Read the model definition and answer for the solid it produces. Units are mm, in the model's axes. Give positions to 0.01 mm unless a question says otherwise; leave off trailing zeros. Write each loop counter-clockwise with the first axis right and the second up, starting at its lowest first coordinate (ties: lowest second). Pieces come first, ordered by that corner, then holes. Notation, with made-up numbers: M 24,80 L 48,80 A18 cw 48,102 Z; hole C 45.5,25 d6. An arc over 180 degrees is marked long. Use a Markdown table: item, result. Add a question column.
Item 1: A cutting plane is placed at B-B on x = 72.5. Determine the outline of the cut face in (y, z).
Item 2: A cutting plane is placed at A-A on y = 6.5. Determine the outline of the cut face in (x, z), then the cut area to 3 significant figures.
Item 3: Given P1, Ø3.5, axis at x = -258, z = 0, coming from the +Y side, flat-ended and moving along its own axis, determine where the tip first touches the part or whether it passes through.
Item 4: Consider probe 1 along Z at (x, y) = (290, 1.1); probe 2 along X at (y, z) = (9.5, -5.5); probe 3 along X at (y, z) = (8.25, 15). Determine where each line is inside the solid, lowest interval first. Write a range as [from, to].
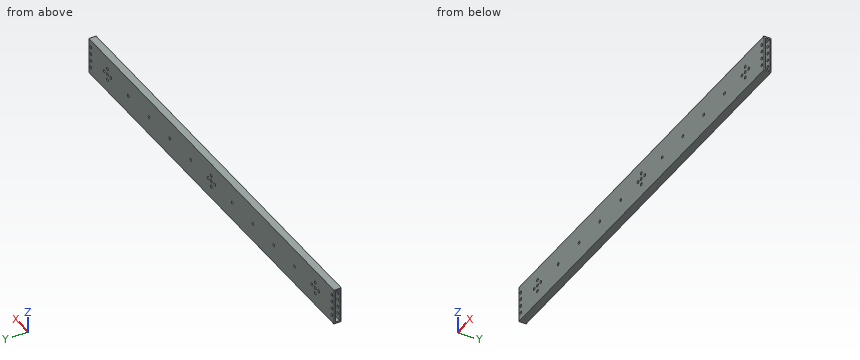
from build123d import *

# Parameters (mm, degrees)
SKETCH_1_W          = 700
SKETCH_1_H          = 50
EXTRUDE_1_DEPTH     = 10
SKETCH_2_R          = 2.05
CUT_EXTRUDE_2_DEPTH = 352.034186369
SKETCH_3_R          = 2.05
CUT_EXTRUDE_3_DEPTH = 352.034186369
SKETCH_4_W          = 46
SKETCH_4_H          = 6
CUT_EXTRUDE_4_DEPTH = 701.51766573
SKETCH_6_W          = 50
SKETCH_6_H          = 10
CUT_EXTRUDE_6_DEPTH = 5
SKETCH_7_R          = 2
CUT_EXTRUDE_7_DEPTH = 347.04912946
SKETCH_8_W          = 50
SKETCH_8_H          = 10
CUT_EXTRUDE_8_DEPTH = 50


with BuildPart() as part:
    # 草图1 → 凸台-拉伸1 (new body)
    with BuildSketch(Plane(origin=(0, 0, 0), x_dir=(1, 0, 0), z_dir=(0, 1, 0))):
        Rectangle(SKETCH_1_W, SKETCH_1_H)
    extrude(amount=EXTRUDE_1_DEPTH)

    # 草图2 → 切除-拉伸2 (cut, through all)
    with BuildSketch(Plane(origin=(0, 10, 0), x_dir=(1, 0, 0), z_dir=(0, 1, 0))):
        with Locations(Location((-300, 0, 0), (0, 0, 270))):
            Circle(SKETCH_2_R)
        with Locations(Location((-250, 0, 0), (0, 0, 270))):
            Circle(SKETCH_2_R)
        with Locations(Location((-200, 0, 0), (0, 0, 270))):
            Circle(SKETCH_2_R)
        with Locations(Location((-150, 0, 0), (0, 0, 270))):
            Circle(SKETCH_2_R)
        with Locations(Location((-100, 0, 0), (0, 0, 270))):
            Circle(SKETCH_2_R)
        with Locations(Location((-50, 0, 0), (0, 0, 270))):
            Circle(SKETCH_2_R)
        with Locations(Location((0, 0, 0), (0, 0, 270))):
            Circle(SKETCH_2_R)
        with Locations(Location((50, 0, 0), (0, 0, 270))):
            Circle(SKETCH_2_R)
        with Locations(Location((100, 0, 0), (0, 0, 270))):
            Circle(SKETCH_2_R)
        with Locations(Location((150, 0, 0), (0, 0, 270))):
            Circle(SKETCH_2_R)
        with Locations(Location((200, 0, 0), (0, 0, 270))):
            Circle(SKETCH_2_R)
        with Locations(Location((250, 0, 0), (0, 0, 270))):
            Circle(SKETCH_2_R)
        with Locations(Location((300, 0, 0), (0, 0, 270))):
            Circle(SKETCH_2_R)
    extrude(amount=-CUT_EXTRUDE_2_DEPTH, mode=Mode.SUBTRACT)

    # 草图3 → 切除-拉伸3 (cut, through all)
    with BuildSketch(Plane(origin=(0, 10, 0), x_dir=(1, 0, 0), z_dir=(0, 1, 0))):
        with Locations(Location((-242, 0, 0), (0, 0, 270))):
            Circle(SKETCH_3_R)
        with Locations(Location((-258, 0, 0), (0, 0, 270))):
            Circle(SKETCH_3_R)
        with Locations(Location((-8, 0, 0), (0, 0, 270))):
            Circle(SKETCH_3_R)
        with Locations(Location((8, 0, 0), (0, 0, 270))):
            Circle(SKETCH_3_R)
        with Locations(Location((242, 0, 0), (0, 0, 270))):
            Circle(SKETCH_3_R)
        with Locations(Location((258, 0, 0), (0, 0, 270))):
            Circle(SKETCH_3_R)
        with Locations(Location((-250, 8, 0), (0, 0, 270))):
            Circle(SKETCH_3_R)
        with Locations(Location((-250, -8, 0), (0, 0, 270))):
            Circle(SKETCH_3_R)
        with Locations(Location((0, 8, 0), (0, 0, 270))):
            Circle(SKETCH_3_R)
        with Locations(Location((0, -8, 0), (0, 0, 270))):
            Circle(SKETCH_3_R)
        with Locations(Location((250, 8, 0), (0, 0, 270))):
            Circle(SKETCH_3_R)
        with Locations(Location((250, -8, 0), (0, 0, 270))):
            Circle(SKETCH_3_R)
    extrude(amount=-CUT_EXTRUDE_3_DEPTH, mode=Mode.SUBTRACT)

    # 草图4 → 切除-拉伸4 (cut, through all)
    with BuildSketch(Plane.ZY.offset(350)):
        with Locations((0, 5)):
            Rectangle(SKETCH_4_W, SKETCH_4_H)
    extrude(amount=-CUT_EXTRUDE_4_DEPTH, mode=Mode.SUBTRACT)

    # 草图6 → 切除-拉伸6 (cut)
    with BuildSketch(Plane(origin=(350, 0, 0), x_dir=(0, 0, -1), z_dir=(1, 0, 0))):
        with Locations((0, 5)):
            Rectangle(SKETCH_6_W, SKETCH_6_H)
    cut_extrude_6 = extrude(amount=-CUT_EXTRUDE_6_DEPTH, mode=Mode.SUBTRACT)

    # 镜向1: 切除-拉伸6 across plane
    add(cut_extrude_6.mirror(Plane(origin=(0, 0, 0), x_dir=(0, 0, 1), z_dir=(1, 0, 0))), mode=Mode.SUBTRACT)

    # 草图7 → 切除-拉伸7 (cut, through all)
    with BuildSketch(Plane(origin=(0, 10, 0), x_dir=(1, 0, 0), z_dir=(0, 1, 0))):
        with Locations(Location((340, 15, 0), (0, 0, 270))):
            Circle(SKETCH_7_R)
        with Locations(Location((340, 5, 0), (0, 0, 270))):
            Circle(SKETCH_7_R)
        with Locations(Location((340, -5, 0), (0, 0, 270))):
            Circle(SKETCH_7_R)
        with Locations(Location((340, -15, 0), (0, 0, 270))):
            Circle(SKETCH_7_R)
        with Locations(Location((290, 5, 0), (0, 0, 270))):
            Circle(SKETCH_7_R)
        with Locations(Location((290, 15, 0), (0, 0, 270))):
            Circle(SKETCH_7_R)
        with Locations(Location((290, -5, 0), (0, 0, 270))):
            Circle(SKETCH_7_R)
        with Locations(Location((290, -15, 0), (0, 0, 270))):
            Circle(SKETCH_7_R)
    cut_extrude_7 = extrude(amount=-CUT_EXTRUDE_7_DEPTH, mode=Mode.SUBTRACT)

    # 镜向2: 切除-拉伸7 across plane
    add(cut_extrude_7.mirror(Plane(origin=(0, 0, 0), x_dir=(0, 0, 1), z_dir=(1, 0, 0))), mode=Mode.SUBTRACT)

    # 草图8 → 切除-拉伸8 (cut)
    with BuildSketch(Plane(origin=(345, 0, 0), x_dir=(0, 0, -1), z_dir=(1, 0, 0))):
        with Locations((0, 5)):
            Rectangle(SKETCH_8_W, SKETCH_8_H)
    cut_extrude_8 = extrude(amount=-CUT_EXTRUDE_8_DEPTH, mode=Mode.SUBTRACT)

    # 镜向3: 切除-拉伸8 across plane
    add(cut_extrude_8.mirror(Plane(origin=(0, 0, 0), x_dir=(0, 0, 1), z_dir=(1, 0, 0))), mode=Mode.SUBTRACT)


solid = part.part
Filled in:
| question | item | result |
|---|---|---|
| 1 | outline | M 0,-25 L 10,-25 L 10,25 L 0,25 Z; hole M 2,-23 L 8,-23 L 8,23 L 2,23 Z |
| 2 | outline | M -295,-25 L 295,-25 L 295,-23 L -295,-23 Z; M -295,23 L 295,23 L 295,25 L -295,25 Z |
| 2 | area | 2,360 mm² |
| 3 | P1 | through |
| 4 | probe 1 | [-25, -17], [-13, -7], [-3, 3], [7, 13], [17, 25] |
| 4 | probe 2 | [-295, -291.94], [-288.06, 288.06], [291.94, 295] |
| 4 | probe 3 | [-295, -292], [-288, 288], [292, 295] |
